Work out the finished part from the listing and answer in its coordinate system (mm). Face numbers are marked on the shaded views. Round coordinates to 2 decimals unless told otherwise and drop trailing zeros. Order: outer loops, then holes, each group sorted by start corner. A loop starts at its lowest first (then second) coordinate and runs counter-clockwise, first axis right, second up. Notation, with made-up numbers: M 14,57 L 49,57 A22 cw 49,67 Z; hole C 14.5,-19.75 d7. An arc over 180 degrees is marked long. Answer as a JSON object with one key per item and string values. Group by question number.
from build123d import *

# Parameters (mm, degrees)
SKETCH1_W                                           = 115
SKETCH1_H                                           = 45
BOSS_EXTRUDE1_DEPTH                                 = 5
CUT_EXTRUDE1_REACH                                  = 119.287
SKETCH2_R                                           = 9.8171
CSK_FOR_M2_COUNTERSUNK_FLAT_HEAD_SCREW1_D           = 2.4
CSK_FOR_M2_COUNTERSUNK_FLAT_HEAD_SCREW1_CSINK_D     = 5.4
CSK_FOR_M2_COUNTERSUNK_FLAT_HEAD_SCREW1_CSINK_ANGLE = 90
SKETCH13_W                                          = 52
SKETCH13_H                                          = 45
BOSS_EXTRUDE4_DEPTH                                 = 6
CHAMFER2_SIZE                                       = 6
M3_TAPPED_HOLE1_D                                   = 2.5
CHAMFER1_SIZE                                       = 3


with BuildPart() as part:
    # Sketch1 → Boss-Extrude1 (new body)
    with BuildSketch(Plane(origin=(0, 0, 0), x_dir=(1, 0, 0), z_dir=(0, 1, 0))):
        with Locations((57.5, 0)):
            Rectangle(SKETCH1_W, SKETCH1_H)
    extrude(amount=BOSS_EXTRUDE1_DEPTH)

    # Sketch2 → Cut-Extrude1 (cut, up to next)
    with BuildSketch(Plane(origin=(0, 5, 0), x_dir=(1, 0, 0), z_dir=(0, 1, 0)), mode=Mode.PRIVATE) as cut_extrude1_sk1:
        with Locations(Location((22.5, 0, 0), (0, 0, 270))):
            Circle(SKETCH2_R)
    cut_extrude1_tool1 = extrude(cut_extrude1_sk1.sketch, amount=-CUT_EXTRUDE1_REACH, mode=Mode.PRIVATE) & part.part
    add(cut_extrude1_tool1.solids().sort_by_distance((22.5, 5, 0))[0], mode=Mode.SUBTRACT)

    # CSK for M2 Countersunk Flat Head Screw1 (through all)
    with Locations(Plane(origin=(0, 5, 0), x_dir=(1, 0, 0), z_dir=(0, 1, 0))):
        with Locations((4, -18.5), (41, -18.5), (41, 5), (4, 5)):
            CounterSinkHole(CSK_FOR_M2_COUNTERSUNK_FLAT_HEAD_SCREW1_D / 2, CSK_FOR_M2_COUNTERSUNK_FLAT_HEAD_SCREW1_CSINK_D / 2, counter_sink_angle=CSK_FOR_M2_COUNTERSUNK_FLAT_HEAD_SCREW1_CSINK_ANGLE)

    # Sketch13 → Boss-Extrude4 (add)
    with BuildSketch(Plane(origin=(0, 5, 0), x_dir=(1, 0, 0), z_dir=(0, 1, 0))):
        with Locations((89, 0)):
            Rectangle(SKETCH13_W, SKETCH13_H)
    extrude(amount=BOSS_EXTRUDE4_DEPTH)

    # Chamfer2
    chamfer2_edges = [part.edges().sort_by_distance(p)[0] for p in [
        (63, 11, 0),
    ]]
    chamfer(chamfer2_edges, length=CHAMFER2_SIZE - 0.0001)  # a hair under: the kernel refuses the full size

    # M3 Tapped Hole1 (through all)
    with Locations(Plane(origin=(0, 11, 0), x_dir=(1, 0, 0), z_dir=(0, 1, 0))):
        with Locations((83, 16), (111, 16), (83, -16), (111, -16)):
            Hole(M3_TAPPED_HOLE1_D / 2)

    # Chamfer1
    chamfer1_edges = [part.edges().sort_by_distance(p)[0] for p in [
        (115, 5.5, -22.5),
        (115, 5.5, 22.5),
    ]]
    chamfer(chamfer1_edges, length=CHAMFER1_SIZE)


solid = part.part
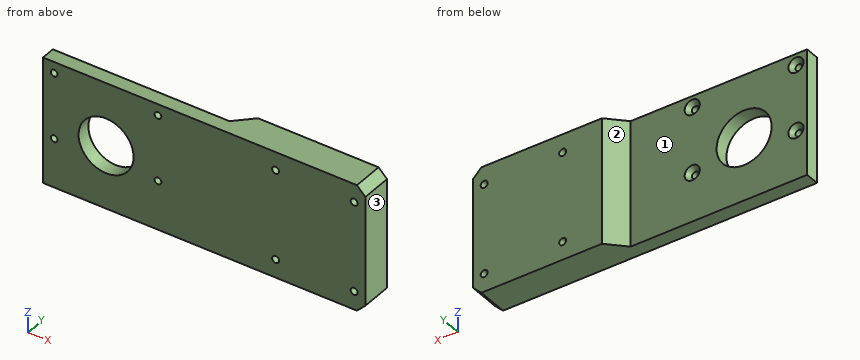
Item 1: Consider L1, parallel to X at y = 4.5, z = -16; L2, parallel to Z at x = 4, y = 0.85; L3, parallel to Z at x = 111, y = 8. Determine where each line is inside the solid, lowest interval first.
Item 2: Find section C-C (x = 22.5). Give the vertices of the cut face in (y, z).
Item 3: Find section A-A (y = 2.5). Give the number of separate pieces and of enclosed holes in the cut face, and give its area (3 significant figures).
Item 4: The mould has two halves that part along X. Classify the marked faces 1, 2 and 3: +X half, -X half, draft (parallel to the pull), parting line (faces both ways), or undercut.
Item 5: Each of these flat-tipped pins is pushed along its axis until it touches: pin 1 (3 mm diameter, centred on x = 111, z = 16, fed in from +Y); pin 2 (3 mm diameter, centred on x = 4, z = -5, fed in from +Y). Where does it stop, or does it pass through?
Item 6: Find section B-B (x = 111). Give the vertices of the cut face in (y, z).
Responses:
{
 "1": {"L1": "x = 0 to 81.75, 84.25 to 109.75, 112.25 to 115", "L2": "z = -22.5 to -6.2, -3.8 to 17.3, 19.7 to 22.5", "L3": "z = -22.5 to -17.25, -14.75 to 14.75, 17.25 to 22.5"},
 "2": {"outline": "M 0,-22.5 L 5,-22.5 L 5,-9.82 L 0,-9.82 Z; M 0,9.82 L 5,9.82 L 5,22.5 L 0,22.5 Z"},
 "3": {"separate pieces": "1", "enclosed holes": "9", "area": "4,830 mm^2"},
 "4": {"face 1": "draft", "face 2": "-X half", "face 3": "+X half"},
 "5": {"pin 1": "stops at y = 11", "pin 2": "stops at y = 3.8"},
 "6": {"outline": "M 0,-22.5 L 11,-22.5 L 11,-17.25 L 0,-17.25 Z; M 0,-14.75 L 11,-14.75 L 11,14.75 L 0,14.75 Z; M 0,17.25 L 11,17.25 L 11,22.5 L 0,22.5 Z"}
}
